Part print with two shaded views. Sizes in mm from the minimum x, y, z corner. Round coordinates to 2 decimals unless told otherwise and drop trailing zeros. Write each loop counter-clockwise with the first axis right and the second up, starting at its lowest first coordinate (ties: lowest second). Pieces come first, ordered by that corner, then holes. Notation, with made-up numbers: M 21,17 L 80,17 A26 cw 80,50 Z; hole C 21,-16.75 d8. An arc over 180 degrees is marked long. Use one line per item in the form item = value. Start each with the question number.
Item 1: Flat gauge pins, fed straight in: pin 1 Ø1.6 at (x, z) = (2, 1.5) entering from -Y (3 decimals); pin 2 Ø1.6 at (x, z) = (92.5, 1.5) entering from +Y; pin 3 Ø1.6 at (y, z) = (53.5, 1.5) entering from +X (3 decimals). Where does each tip first touch, or does it go through?
Item 2: Cut at A-A, the plane x = 111. Give the cut face in (y, z) (3 decimals).
Item 3: Probe L1, parallel to Y at x = 57, z = 0.95; L2, parallel to X at y = 97, z = 1.55 (3 decimals); L3, parallel to Y at x = 23, z = 2.35. List the from-to ranges inside material, lowest first.
Item 4: Cut at B-B, the plane y = 59. Give the cut face in (x, z) (3 decimals).
Item 5: Cut at D-D, the plane z = 2. Give the cut face in (x, y) (3 decimals).
Item 6: Cut at C-C, the plane x = 87. Give the cut face in (y, z) (3 decimals).
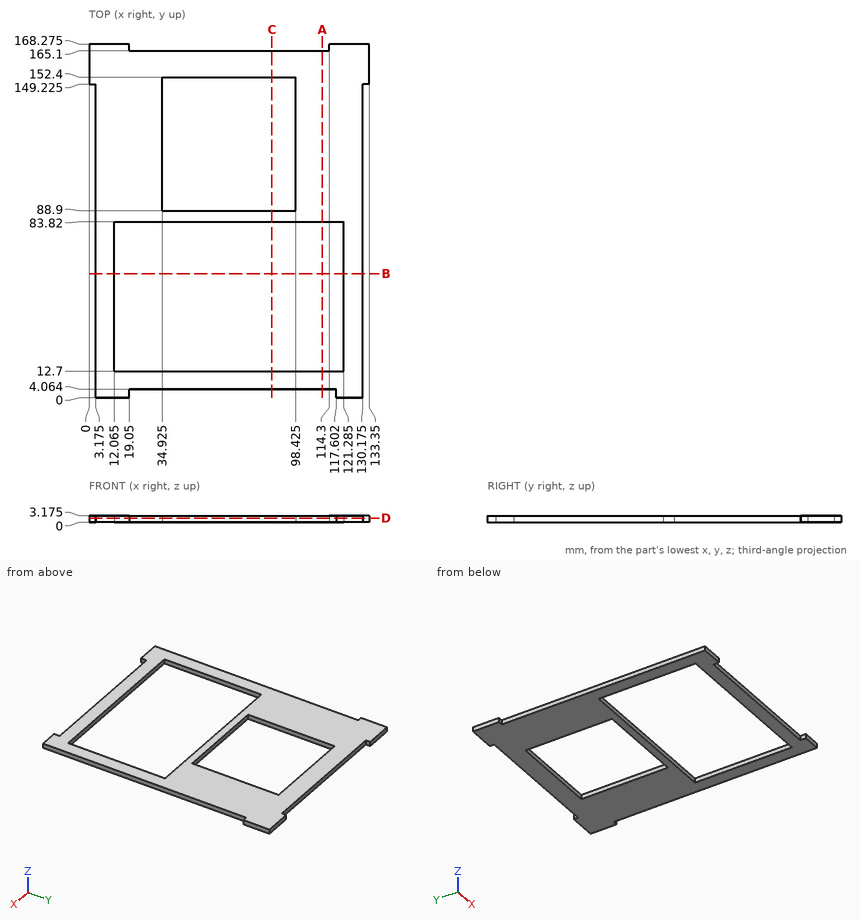
Model answer:
q1.pin_1 = 149.225
q1.pin_2 = 165.1
q1.pin_3 = 130.175
q2.outline = M 4.064,0 L 12.7,0 L 12.7,3.175 L 4.064,3.175 Z; M 83.82,0 L 165.1,0 L 165.1,3.175 L 83.82,3.175 Z
q3.L1 = 4.06 to 12.7, 83.82 to 88.9, 152.4 to 165.1
q3.L2 = 3.175 to 34.925, 98.425 to 130.175
q3.L3 = 4.06 to 12.7, 83.82 to 165.1
q4.outline = M 3.175,0 L 12.065,0 L 12.065,3.175 L 3.175,3.175 Z; M 121.285,0 L 130.175,0 L 130.175,3.175 L 121.285,3.175 Z
q5.outline = M 0,149.225 L 3.175,149.225 L 3.175,0 L 19.05,0 L 19.05,4.064 L 117.602,4.064 L 117.602,0 L 130.175,0 L 130.175,149.225 L 133.35,149.225 L 133.35,168.275 L 114.3,168.275 L 114.3,165.1 L 19.05,165.1 L 19.05,168.275 L 0,168.275 Z; hole M 12.065,12.7 L 121.285,12.7 L 121.285,83.82 L 12.065,83.82 Z; hole M 34.925,88.9 L 98.425,88.9 L 98.425,152.4 L 34.925,152.4 Z
q6.outline = M 4.064,0 L 12.7,0 L 12.7,3.175 L 4.064,3.175 Z; M 83.82,0 L 88.9,0 L 88.9,3.175 L 83.82,3.175 Z; M 152.4,0 L 165.1,0 L 165.1,3.175 L 152.4,3.175 Z
